```python
from build123d import *

# Parameters (mm, degrees)
BOSS_EXTRUDE1_DEPTH = 8
SKETCH2_R           = 1.7
CUT_EXTRUDE1_DEPTH  = 19.867962264
CHAMFER1_SIZE       = 1
FILLET1_R           = 1


with BuildPart() as part:
    # Sketch1 → Boss-Extrude1 (new body)
    with BuildSketch(Plane(origin=(0, 0, 0), x_dir=(1, 0, 0), z_dir=(0, 1, 0))):
        with BuildLine():
            Line((-16, 0), (-8.485281374, 0))
            ThreePointArc((-8.485281374, 0), (-6.753230567, -0.550510257), (-5.656854249, -2))
            ThreePointArc((-5.656854249, -2), (-3.464101615, -4.898979486), (0, -6))
            Line((0, -6), (0, -8))
            ThreePointArc((0, -8), (-4.618802154, -6.531972647), (-7.542472333, -2.666666667))
            ThreePointArc((-7.542472333, -2.666666667), (-7.907931105, -2.183503419), (-8.485281374, -2))
            Line((-8.485281374, -2), (-16, -2))
            Line((-16, -2), (-16, 0))
        make_face()
    extrude(amount=BOSS_EXTRUDE1_DEPTH)

    # Sketch2 → Cut-Extrude1 (cut, through all)
    with BuildSketch(Plane.XY.offset(2)):
        with Locations((-12, 4)):
            Circle(SKETCH2_R)
    extrude(amount=-CUT_EXTRUDE1_DEPTH, mode=Mode.SUBTRACT)

    # Chamfer1
    chamfer1_edges = [part.edges().sort_by_distance(p)[0] for p in [
        (-16, 0, 1),
        (-16, 8, 1),
    ]]
    chamfer(chamfer1_edges, length=CHAMFER1_SIZE)

    # Fillet1
    fillet1_edges = [part.edges().sort_by_distance(p)[0] for p in [
        (-16, 4, 0),
        (-16, 4, 2),
        (-15.5, 0.5, 0),
        (-15.5, 0.5, 2),
        (-15.5, 7.5, 0),
        (-15.5, 7.5, 2),
        (-15, 8, 1),
        (-15, 0, 1),
    ]]
    fillet(fillet1_edges, radius=FILLET1_R - 0.0001)  # a hair under: the kernel refuses the full size

    # Mirror1: part across plane


with BuildPart() as part_1:
    add(part.part)
    add(part.part.mirror(Plane(origin=(0, 8, 6), x_dir=(0, 0, 1), z_dir=(-1, 0, 0))))


solid = part_1.part
```
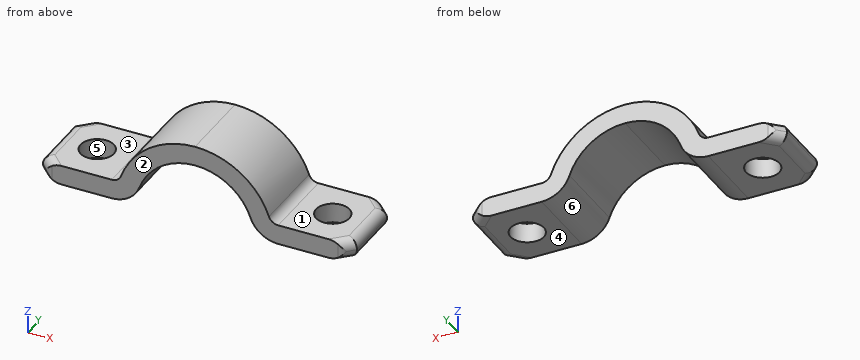
For this review, take the finished solid that the model builds, in its own axes (mm). Face numbers are marked on the shaded views. A direction names the side the tool comes from. Coordinates: 2 decimals unless noted, no trailing zeros. Write each loop counter-clockwise with the first axis right and the second up, starting at its lowest first coordinate (ties: lowest second). Pieces come first, ordered by that corner, then holes.
(1) For pin 1 Ø1 at (y, z) = (4.5, 4) entering from +X; pin 2 Ø1.5 at (y, z) = (1.5, 4) entering from +X; pin 3 Ø4.5 at (x, y) = (-12, 4) entering from +Z, all flat-tipped, find the tip position at first contact; note any pin that passes through.
(2) Add section A-A on y = 4. Count the separate pieces of the cut face and the enclosed holes in it, then the cut area to 3 significant figures.
(3) Wall thickness on probe 1 along Y at (x, z) = (12, 1.1); probe 2 along X at (y, z) = (3, 3.5); probe 3 along X at (y, z) = (3, 3): over which ranges is each line inside the solid? List them lowest first.
(4) Add section D-D on x = 5. Give the boundary of the cut face in (y, z) (3 decimals).
(5) Add section B-B on x = -12. Give the boundary of the cut face in (y, z).
(6) Tool access review of the marked faces 1, 2 and 3: name each direction out of +Z, -Z, +X, -X, +Y, -Y from which nothing blocks a thin tool from reaching the whole face with its end or side.
(7) Add section C-C on z = 4.75. Give the boundary of the cut face in (x, y), then the cut area to 3 significant figures.
(8) The part is to be moulded in two halves that separate along X. For the marked faces 4, 5 and 6, say which applies: +X half, -X half, draft (parallel to the pull), parting line (faces both ways), or undercut.
Answer sheet:
1. pin 1: stops at x = 7.19
1. pin 2: stops at x = 7.31
1. pin 3: stops at z = 2
2. separate pieces: 3
2. enclosed holes: 0
2. area: 59.9 mm2
3. probe 1: y = 0 to 2.3, 5.7 to 8
3. probe 2: x = -7.19 to -4.87, 4.87 to 7.19
3. probe 3: x = -7.42 to -5.2, 5.2 to 7.42
4. outline: (0, 3.317) - (8, 3.317) - (8, 6.245) - (0, 6.245) - close
5. outline: (0, 0) - (2.3, 0) - (2.3, 2) - (0, 2) - close; (5.7, 0) - (8, 0) - (8, 2) - (5.7, 2) - close
6. face 1: +Z, +X, +Y, -Y
6. face 2: +Z, -Z, +X, -X, -Y
6. face 3: +Z, -X, +Y, -Y
7. outline: (-6.44, 0) - (-3.67, 0) - (-3.67, 8) - (-6.44, 8) - close; (3.67, 0) - (6.44, 0) - (6.44, 8) - (3.67, 8) - close
7. area: 44.3 mm2
8. face 4: draft
8. face 5: undercut
8. face 6: undercut
